Could you check a few things on this model? Use its own coordinates, in mm. A direction names the side the tool comes from. Give positions to 0.01 mm unless a question says otherwise; leave off trailing zeros. Loops run counter-clockwise (first coordinate to the right, second up) from the corner with the lowest first, then second, coordinate; pieces in that order, holes last. Notation, with made-up numbers: (61.25, 31) - (66.25, 31) arc R29 ccw to (66.25, 54) - close; hole circle Ø8 at (20.25, 1.5). An arc over 180 degrees is marked (long way). Answer in a Markdown table with one row per item. Add a question column.
```python
from build123d import *

# Parameters (mm, degrees)
SKETCH1_R                      = 44.675
BOSS_EXTRUDE2_DEPTH            = 6.35
M5_CLEARANCE_HOLE2_D           = 5.5
M5_CLEARANCE_HOLE2_CSINK_D     = 5.55
M5_CLEARANCE_HOLE2_CSINK_ANGLE = 90
CIRPATTERN1_COUNT              = 6
SKETCH13_R                     = 44.675
SKETCH13_R_2                   = 39.675
BOSS_EXTRUDE4_DEPTH            = 21.65


with BuildPart() as part:
    # Sketch1 → Boss-Extrude2 (new body)
    with BuildSketch(Plane(origin=(0, 0, 0), x_dir=(1, 0, 0), z_dir=(0, 1, 0))):
        with Locations(Location((0, 0, 0), (0, 0, 270))):
            Circle(SKETCH1_R)
    extrude(amount=BOSS_EXTRUDE2_DEPTH)

    # M5 Clearance Hole2 (through all)
    with Locations(Plane(origin=(0, 6.35, 0), x_dir=(1, 0, 0), z_dir=(0, 1, 0))):
        with Locations((0, 13.5)):
            m5_clearance_hole2 = CounterSinkHole(M5_CLEARANCE_HOLE2_D / 2, M5_CLEARANCE_HOLE2_CSINK_D / 2, counter_sink_angle=M5_CLEARANCE_HOLE2_CSINK_ANGLE)

    # CirPattern1: M5 Clearance Hole2 ×6 about axis
    cirpattern1_axis = Axis((0, 0, 0.0522889), (0, 1, 0))
    for i in range(1, CIRPATTERN1_COUNT):
        add(m5_clearance_hole2.rotate(cirpattern1_axis, i * 360 / CIRPATTERN1_COUNT), mode=Mode.SUBTRACT)

    # Sketch13 → Boss-Extrude4 (add)
    # profile 1 of 4: a face of its own
    with BuildSketch(Plane(origin=(0, 6.35, 0), x_dir=(1, 0, 0), z_dir=(0, 1, 0))):
        with Locations(Location((0, 0, 0), (0, 0, 270))):
            Circle(SKETCH13_R)
        with Locations(Location((0, 0, 0), (0, 0, 90))):
            Circle(SKETCH13_R_2, mode=Mode.SUBTRACT)
    # profile 2 of 4: a face of its own
    with BuildSketch(Plane(origin=(0, 6.35, 0), x_dir=(1, 0, 0), z_dir=(0, 1, 0))):
        with Locations(Location((0, 0, 0), (0, 0, 270))):
            Circle(SKETCH13_R)
        with Locations(Location((0, 0, 0), (0, 0, 90))):
            Circle(SKETCH13_R_2, mode=Mode.SUBTRACT)
    # profile 3 of 4: a face of its own
    with BuildSketch(Plane(origin=(0, 6.35, 0), x_dir=(1, 0, 0), z_dir=(0, 1, 0))):
        with Locations(Location((0, 0, 0), (0, 0, 270))):
            Circle(SKETCH13_R)
        with Locations(Location((0, 0, 0), (0, 0, 90))):
            Circle(SKETCH13_R_2, mode=Mode.SUBTRACT)
    # profile 4 of 4: a face of its own
    with BuildSketch(Plane(origin=(0, 6.35, 0), x_dir=(1, 0, 0), z_dir=(0, 1, 0))):
        with Locations(Location((0, 0, 0), (0, 0, 270))):
            Circle(SKETCH13_R)
        with Locations(Location((0, 0, 0), (0, 0, 90))):
            Circle(SKETCH13_R_2, mode=Mode.SUBTRACT)
    extrude(amount=BOSS_EXTRUDE4_DEPTH)


solid = part.part
```
(1) We'd pull the mould along X, two halves only. Please class faces 3 (the cylindrical face through (44.295, 13.804, -5.816)), 4 (the cylindrical face through (-14.36, 3.12, 6)), 5 (the flat face through (1, 0, -1)), 6 (the flat face through (1, 6.35, -1)): pulls with the +X half, pulls with the -X half, needs draft (parallel to the pull), parting line crosses it, or undercut.
(2) On a 3-axis mill with a long thin cutter (end or side, diameter ignored), from which of +Z, -Z, +X, -X, +Y, -Y can I reach the whole of each face in a straight line? I mean faces 1 (the cylindrical face through (38.73, 17.02, 8.6)), 2 (the cylindrical face through (12.333, 3.118, 9.513)). Say none if no direction works.
(3) Please list where these lines run through material, in increasing order: line 1 (Y direction, x = 3.5, z = -39); line 2 (Z direction, x = -4, y = 25.5); line 3 (Z direction, x = -14, y = 7).
(4) I want a section at B-B on y = 3.5. Please give me the cut outline in (x, z) (3 decimals).
(5) I want a section at A-A on x = 0. Please give me the cut outline in (y, z) (3 decimals).
(6) I want a section at D-D on z = 0. Please give me the cut outline in (x, y) (3 decimals).
(7) I want a section at C-C on z = -13.5. Please give me the cut outline in (x, y) (3 decimals).
(8) For pin 1 Ø12 at (y, z) = (9.5, 8) entering from -X; pin 2 Ø3 at (x, z) = (-14, -18.5) entering from +Y; pin 3 Ø10 at (y, z) = (7, -19.5) entering from -X, each with a flat end and sliding along its axis, tell me the tip position at first contact or that it passes through.
Reported:
| question | item | result |
|---|---|---|
| 1 | face 3 | parting line crosses it |
| 1 | face 4 | undercut |
| 1 | face 5 | needs draft |
| 1 | face 6 | undercut |
| 2 | face 1 | +Y |
| 2 | face 2 | +Y, -Y |
| 3 | line 1 | 0 to 6.35 |
| 3 | line 2 | -44.5 to -39.47, 39.47 to 44.5 |
| 3 | line 3 | -42.42 to -37.12, 37.12 to 42.42 |
| 4 | outline | circle Ø89.35 at (0, 0); hole circle Ø5.5 at (-11.737, -6.724); hole circle Ø5.5 at (-11.737, 6.828); hole circle Ø5.5 at (0, -13.5); hole circle Ø5.5 at (0, 13.605); hole circle Ø5.5 at (11.737, -6.724); hole circle Ø5.5 at (11.737, 6.828) |
| 5 | outline | (0, -44.675) - (28, -44.675) - (28, -39.675) - (6.35, -39.675) - (6.35, -16.275) - (6.325, -16.25) - (0, -16.25) - close; (0, -10.75) - (6.325, -10.75) - (6.35, -10.725) - (6.35, 10.83) - (6.325, 10.855) - (0, 10.855) - close; (0, 16.355) - (6.325, 16.355) - (6.35, 16.38) - (6.35, 39.675) - (28, 39.675) - (28, 44.675) - (0, 44.675) - close |
| 6 | outline | (-44.675, 0) - (44.675, 0) - (44.675, 28) - (39.675, 28) - (39.675, 6.35) - (-39.675, 6.35) - (-39.675, 28) - (-44.675, 28) - close |
| 7 | outline | (-42.586, 0) - (-2.75, 0) - (-2.75, 6.325) - (-2.775, 6.35) - (-37.308, 6.35) - (-37.308, 28) - (-42.586, 28) - close; (2.75, 0) - (42.586, 0) - (42.586, 28) - (37.308, 28) - (37.308, 6.35) - (2.775, 6.35) - (2.75, 6.325) - close |
| 8 | pin 1 | x = -44.63 |
| 8 | pin 2 | y = 6.35 |
| 8 | pin 3 | x = -42.26 |
